Source: CAD feature listing. Evaluate the final solid. Frame: model axes, mm. Face numbers are marked on the shaded views. A direction names the side the tool comes from. Coordinates: 2 decimals unless noted, no trailing zeros. Write each loop counter-clockwise with the first axis right and the second up, starting at its lowest first coordinate (ties: lowest second). Pieces come first, ordered by that corner, then holes. Notation, with made-up numbers: (-28, 32) -> (23, 32) arc R19 ccw to (23, 47) -> close; hole circle Ø6 at (44.5, 17). An arc over 180 degrees is marked (long way). Write item = value, one per line.
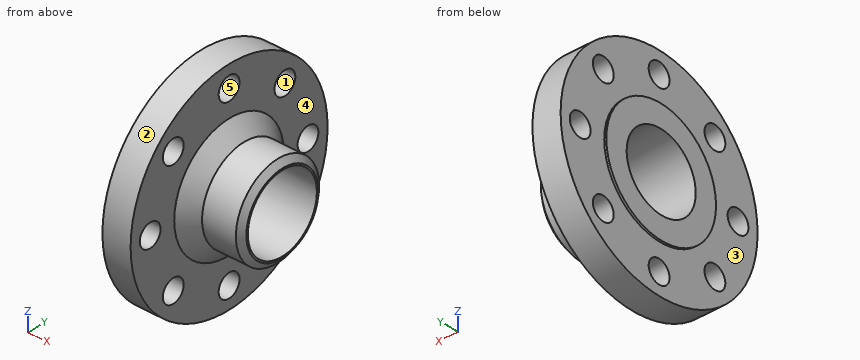
Autodesk Inventor part; units mm, degrees
ref_plane "YZ Plane" through (0, 0, 0) normal (1, 0, 0) x (0, 1, 0)
ref_plane "XZ Plane" through (0, 0, 0) normal (0, 1, 0) x (-1, 0, 0)
ref_plane "XY Plane" through (0, 0, 0) normal (0, 0, 1) x (1, 0, 0)
sketch "Sketch1" plane through (0, 0, 0) normal (0, 0, 1) x (1, 0, 0)
  line L0 (0, 0) -> (109.4884, 0)
  line L1 (0, 36.83) -> (0, 58.5)
  line L2 (0, 58.5) -> (2, 58.5)
  line L3 (2, 58.5) -> (2, 105)
  line L4 (2, 105) -> (29, 105)
  line L5 (29, 105) -> (29, 58.5)
  line L6 (29, 58.5) -> (43.05, 44.45)
  line L7 (43.05, 44.45) -> (75.3807, 44.45)
  line L8 (75.3807, 44.45) -> (80, 38.43)
  line L9 (80, 38.43) -> (80, 36.83)
  line L10 (80, 36.83) -> (0, 36.83)
  point P0 (0, 47.665)
  dimension "d5" = 2
  dimension "d6" = 210
  dimension "d7" = 27
  dimension "d8" = 117
  dimension "d9" = 45
  dimension "d10" = 78
  dimension "d28" = 73.66
  dimension "d29" = 88.9
  dimension "d30" = 37.5
  dimension "d31" = 1.6
revolve "Revolution1" add sketch "Sketch1" angle 360 about axis through (0, 0, 0) along (1, 0, 0)
sketch "Sketch2" plane through (2, 0, 0) normal (-1, 0, 0) x (0, 0, 1)
  point P0 (0, 0)
  point P1 (0, 84.14)
  dimension "d12" = 84.14
hole "Hole1" at (2, 84.14, 0) direction (1, 0, 0) diameter 22.225 end up to surface
pattern_circular "Circular Pattern1" count 8 over 360 about axis through (15.5, 0, 0) along (1, 0, 0) of "Hole1"
properties part number "Flange 3 in" material "ASTM A105 Gr.B"
1) Cut plane D-D, the plane y = -63. Output: boundary loops of the cut face in (x, z), and give its area (3 significant figures).
Answer block:
outline = (2, -84) -> (29, -84) -> (29, -70.04) -> (2, -70.04) -> close; (2, -48.95) -> (29, -48.95) -> (29, 48.95) -> (2, 48.95) -> close; (2, 70.04) -> (29, 70.04) -> (29, 84) -> (2, 84) -> close
area = 3,400 mm2
2) Reachability of the marked faces 4 and 5 from +Z, -Z, +X, -X, +Y, -Y: full face, straight path, thin tool, end or side. Return the list, or none.
Answer block:
face_4 = +X
face_5 = +X, -X
3) Cut plane A-A, the plane z = -79. Output: boundary loops of the cut face in (x, y), and give its area (3 significant figures).
Answer block:
outline = (2, -69.17) -> (29, -69.17) -> (29, -9.85) -> (2, -9.85) -> close; (2, 9.85) -> (29, 9.85) -> (29, 69.17) -> (2, 69.17) -> close
area = 3,200 mm2
4) Cut plane B-B, the plane y = -90. Output: boundary loops of the cut face in (x, z), and give its area (3 significant figures).
Answer block:
outline = (2, -54.08) -> (29, -54.08) -> (29, -9.44) -> (2, -9.44) -> close; (2, 9.44) -> (29, 9.44) -> (29, 54.08) -> (2, 54.08) -> close
area = 2,410 mm2
5) Cut plane C-C, the plane x = 19.5. Give the number of separate pieces and of enclosed holes in the cut face, and give its area (3 significant figures).
Answer block:
separate_pieces = 1
enclosed_holes = 9
area = 27,300 mm2
6) Material intervals for probe 1 along Z at (x, y) = (19, 0); probe 2 along Z at (x, y) = (25.5, -54); probe 3 along X at (y, z) = (-85.5, 38), sorted ascending. Write a range as [from, to].
Answer block:
probe_1 = [-105, -95.25], [-73.03, -36.83], [36.83, 73.03], [95.25, 105]
probe_2 = [-90.05, -69.15], [-49.84, 49.84], [69.15, 90.05]
probe_3 = [2, 29]
7) Pull-direction query (Z, two-part tool) for the marked faces 1, 2 and 3; classes: +Z half, -Z half, draft (parallel to the pull), parting line (faces both ways), or undercut.
Answer block:
face_1 = undercut
face_2 = parting line
face_3 = draft
8) First-contact query: pin 1 Ø18 at (y, z) = (-59.5, 59.5) entering from -X; pin 2 Ø4 at (x, y) = (23.5, 68) entering from -Z; pin 3 Ø5 at (x, z) = (30.5, -22) entering from -Y; pin 4 Ø12 at (x, y) = (23.5, 68.5) entering from -Z. Flat tips, straight axial feed; report the tip coordinate or a pass-through.
Answer block:
pin_1 = through
pin_2 = -81.66
pin_3 = -103.08
pin_4 = -84.37
